Could you check a few things on this model? Use its own coordinates, in mm. Face numbers are marked on the shaded views. Coordinates: 2 decimals unless noted, no trailing zeros. Write each loop counter-clockwise with the first axis right and the second up, starting at its lowest first coordinate (ties: lowest second). Pieces come first, ordered by that corner, then holes.
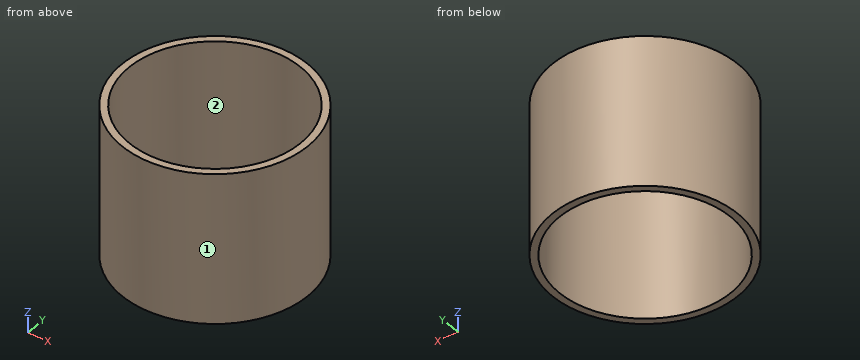
```python
from build123d import *

# Parameters (mm, degrees)
CYLINDER011_R     = 12
CYLINDER011_DEPTH = 21
CYLINDER010_R     = 13
CYLINDER010_DEPTH = 21


with BuildPart() as cylinder006:
    # Cylinder011 → Cylinder011 (new body)
    with BuildSketch(Plane.XY):
        Circle(CYLINDER011_R)
    extrude(amount=CYLINDER011_DEPTH)


with BuildPart() as cut006:
    # Cylinder010 → Cylinder010 (new body)
    with BuildSketch(Plane.XY):
        Circle(CYLINDER010_R)
    extrude(amount=CYLINDER010_DEPTH)

    # Cut006: cut Cylinder006
    add(cylinder006.part, mode=Mode.SUBTRACT)


with BuildPart() as cut006_1:
    # Cut006 placement: moved
    add(cut006.part.moved(Location((0, 0, 21))))


solid = cut006_1.part
```
1. If we mould it in two halves opening along X, with no side actions, what happens to the marked faces 1 and 2? For each: pulls with the +X half, pulls with the -X half, needs draft (parallel to the pull), parting line crosses it, or undercut.
Verdict:
face 1: parting line crosses it
face 2: undercut
2. I want a section at C-C on z = 34. Please give me the cut outline in (x, y), plus the area to 3 significant figures.
Verdict:
outline: circle Ø26 at (0, 0); hole circle Ø24 at (0, 0)
area: 78.5 mm2
3. Please list where these lines run through material, in increasing order: line 1 along Y through (x, z) = (0, 31); line 2 along X through (y, z) = (-2.5, 25.5).
Verdict:
line 1: y = -13 to -12, 12 to 13
line 2: x = -12.76 to -11.74, 11.74 to 12.76
4. For pin 1 (10 mm diameter, centred on x = -6.5, y = 0, fed in from -Z); pin 2 (12 mm diameter, centred on y = -2, z = 36.5, fed in from +X); pin 3 (3 mm diameter, centred on x = 5, z = 27, fed in from -Y); pin 4 (10 mm diameter, centred on y = 8.5, z = 30.5, fed in from -X), each with a flat end and sliding along its axis, tell me the tip position at first contact or that it passes through.
Verdict:
pin 1: passes through
pin 2: stops at x = 13
pin 3: stops at y = -12.52
pin 4: stops at x = -12.52
5. I want a section at A-A on y = 0. Please give me the cut outline in (x, z), plus the area to 3 significant figures.
Verdict:
outline: (-13, 21) - (-12, 21) - (-12, 42) - (-13, 42) - close; (12, 21) - (13, 21) - (13, 42) - (12, 42) - close
area: 42.0 mm2
